Input: part model. Units: mm. Frame: model coordinates. Face numbers are marked on the shaded views. A direction names the side the tool comes from. Coordinates: 2 decimals unless noted, no trailing zeros. Loops run counter-clockwise (first coordinate to the right, second up) from the corner with the lowest first, then second, coordinate; pieces in that order, holes last. Notation, with made-up numbers: (-0.5, -4) - (5.5, -4) arc R6 ccw to (5.5, 2) - close; hole circle Ø9 at (-14, -29). An arc over 180 degrees is marked (long way). Use a Markdown table: item, result. Add a question column.
1. Section query C-C on x = 0. Return the cut outline in (y, z) (3 decimals), then the cut area to 3 significant figures.
2. Access query for the marked faces 1 and 2. Directions: +Z, -Z, +X, -X, +Y, -Y. A direction counts if a zero-diameter tool reaches every point of the face in a straight line with its end or side. Return the directions, or none.
3. Section query A-A on z = 14.75. Return the cut outline in (x, y) (3 decimals), then the cut area to 3 significant figures.
4. Contact query for flat-ended pins moving along their axis: P1, Ø3, axis at y = -8.5, z = 18, coming from the -X side; P2, Ø6, axis at x = -8.5, z = 13.5, coming from the +Y side; P3, Ø12, axis at x = 0, y = 0, coming from the +Z side; P4, Ø2.5, axis at x = -9.5, z = 6, coming from the -Y side (3 decimals). Output: stop coordinate, or through.
5. Section query D-D on y = -8.75. Return the cut outline in (x, z) (3 decimals), then the cut area to 3 significant figures.
6. Section query B-B on z = 7. Return the cut outline in (x, y) (3 decimals), then the cut area to 3 significant figures.
7. Draft query along X for the marked faces 3, 4 and 5. Return one class per face: released by +X, released by -X, zero draft, split by the parting line, or undercut.
8. Ray query, L1, parallel to X at y = -3.75, z = 18 (3 decimals); L2, parallel to Y at x = -4.75, z = 3; L3, parallel to X at y = -2.25, z = 15 (3 decimals). Return the intervals inside material, ascending. Write a range as [from, to].
```python
from build123d import *

# Parameters (mm, degrees)
F1_DEPTH    = 20
F2_R        = 1.25
F3_DEPTH    = 6
F4_T2_ANGLE = 359.64


# Not quite as in the source:
# - a fillet or chamfer that OpenCascade refuses, or shapes differently, is made with other operations: its cross-section is extruded or revolved along the edge and cut away or added
# - a feature names something its author has since deleted; it is built from what else it names


with BuildPart() as f1:
    # F0 (on Top) → F1 (new body)
    with BuildSketch(Plane.XY):
        with BuildLine():
            Line((11.625, -11.625), (11.625, 0))
            ThreePointArc((11.625, 0), (0, 11.625), (-11.625, 0))
            Line((-11.625, 0), (-11.625, -5.125))
            ThreePointArc((-11.625, -5.125), (-11.3321067812, -5.8321067812), (-10.625, -6.125))
            Line((-10.625, -6.125), (-5.6457948953, -6.125))
            ThreePointArc((-5.6457948953, -6.125), (-4.7314286811, -5.5298881651), (-4.9053627779, -4.4528688525))
            ThreePointArc((-4.9053627779, -4.4528688525), (0.5907863647, 6.598605646), (4.0363377793, -5.2534371921))
            ThreePointArc((4.0363377793, -5.2534371921), (3.6647499446, -5.8516258782), (3.7795709082, -6.5464088438))
            Line((3.7795709082, -6.5464088438), (6.4230217447, -11.125))
            ThreePointArc((6.4230217447, -11.125), (6.7890471485, -11.4910254038), (7.2890471485, -11.625))
            Line((7.2890471485, -11.625), (11.625, -11.625))
        make_face()
    extrude(amount=F1_DEPTH)

    # F2 (on face) → F3 (cut)
    with BuildSketch(Plane.YZ.offset(11.625)):
        with Locations((-4.625, 14.75)):
            Circle(F2_R)
        with Locations((-4.625, 5.25)):
            Circle(F2_R)
    extrude(amount=-F3_DEPTH, mode=Mode.SUBTRACT)

    # F4: chamfer of 2 on 1 edges, made by hand

    # F4_s1 → F4_t2 (revolve, cut)
    with BuildSketch(Plane(origin=(0, 0, 0), x_dir=(0, 0, 1), z_dir=(0.9957308794, -0.0923039315, 0))):
        Polygon((0, 8.625), (2, 6.625), (0, 6.625), align=None)
    revolve(axis=Axis((0, 0, 0), (0, 0, -1)), revolution_arc=F4_T2_ANGLE, mode=Mode.SUBTRACT)


solid = f1.part
```
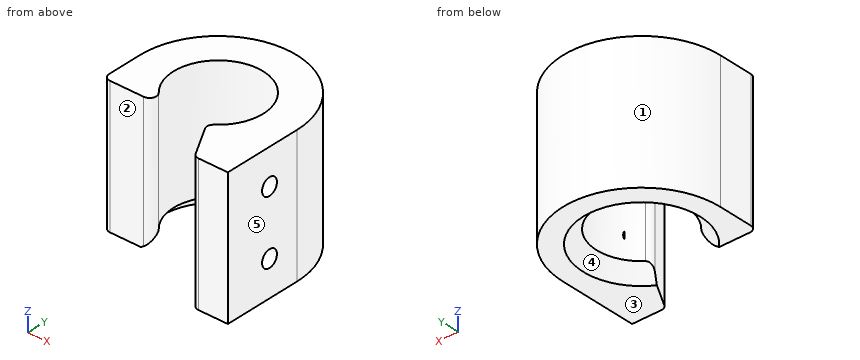
Resolved:
| question | item | result |
|---|---|---|
| 1 | outline | (6.625, 2) - (8.625, 0) - (11.625, 0) - (11.625, 20) - (6.625, 20) - close |
| 1 | area | 98.0 mm² |
| 2 | face 1 | +Z, -Z, +Y |
| 2 | face 2 | +Z, -Z, -X, -Y |
| 3 | outline | (-11.625, -5.125) arc R1 ccw to (-10.625, -6.125) - (-5.646, -6.125) arc R1 ccw to (-4.905, -4.453) arc R6.625 cw (long way) to (5.701, -3.375) - (11.625, -3.375) - (11.625, 0) arc R11.625 ccw to (-11.625, 0) - close; (3.78, -6.546) - (6.423, -11.125) arc R1 ccw to (7.289, -11.625) - (11.625, -11.625) - (11.625, -5.875) - (5.625, -5.875) - (5.625, -3.5) arc R6.625 cw to (4.036, -5.253) arc R1 ccw to start |
| 3 | area | 237 mm² |
| 4 | P1 | x = 4.04 |
| 4 | P2 | y = 10.24 |
| 4 | P3 | through |
| 4 | P4 | y = -6.125 |
| 5 | outline | (5.052, 0) - (11.625, 0) - (11.625, 20) - (5.052, 20) - close |
| 5 | area | 131 mm² |
| 6 | outline | (-11.625, -5.125) arc R1 ccw to (-10.625, -6.125) - (-5.646, -6.125) arc R1 ccw to (-4.905, -4.453) arc R6.625 cw (long way) to (4.036, -5.253) arc R1 ccw to (3.78, -6.546) - (6.423, -11.125) arc R1 ccw to (7.289, -11.625) - (11.625, -11.625) - (11.625, 0) arc R11.625 ccw to (-11.625, 0) - close |
| 6 | area | 252 mm² |
| 7 | face 3 | zero draft |
| 7 | face 4 | undercut |
| 7 | face 5 | released by +X |
| 8 | L1 | [-11.625, -5.462], [5.462, 11.625] |
| 8 | L2 | [-5.57, -4.68], [4.62, 10.61] |
| 8 | L3 | [-11.625, -6.231], [6.231, 11.625] |
